Can you work these out from the model? Positions are in its coordinate system, mm. Face numbers are marked on the shaded views. A direction names the side the tool comes from. Round coordinates to 2 decimals unless told otherwise and drop trailing zeros. Write each loop counter-clockwise with the first axis right and the second up, starting at its lowest first coordinate (ties: lowest second). Pieces come first, ordered by that corner, then holes. Notation, with made-up numbers: (75.5, 79.25) - (124.5, 79.25) arc R16 ccw to (124.5, 99.25) - close; hole circle Ø11 at (57.25, -11). An arc over 180 degrees is marked (long way). One line per item, written item: value. Start each with the question number.
(1) I want a section at B-B on x = 2. List the corners of the cut face in (y, z) for me, plus the area to 3 significant figures.
(2) I want a section at D-D on x = 0. List the corners of the cut face in (y, z) for me, plus the area to 3 significant figures.
(3) I want a section at A-A on z = 4.5. List the corners of the cut face in (x, y) for me (3 decimals), plus the area to 3 significant figures.
(4) Thinking about a two-plate mould opening in Y: for the marked faces 1, 2, 3 and 4, which applies, +Y half, -Y half, draft (parallel to the pull), parting line (faces both ways), or undercut?
(5) I'm going to push flat-ended pins straight in: pin 1 Ø1 at (y, z) = (-5.5, 5) entering from -X; pin 2 Ø5 at (x, y) = (1.5, 4.5) entering from -Z. Where does each tip first touch, or does it pass through?
(6) I want a section at C-C on y = 4.5. List the corners of the cut face in (x, z) for me.
(7) On a 3-axis mill with a long thin cutter (end or side, diameter ignored), from which of +Z, -Z, +X, -X, +Y, -Y can I reach the whole of each face in a straight line? I mean the marked faces 5 and 6. Say none if no direction works.
(8) If I drill on L1, parallel to Y at x = -2.75, z = 2; L2, parallel to Y at x = 2.5, z = 3.5; L3, parallel to X at y = -7, z = 4, over which ranges is the centre line in solid material (lowest first)? Write a range as from..to.
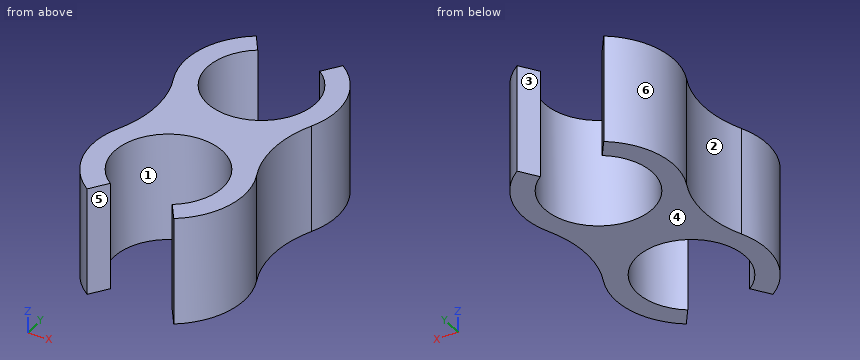
from build123d import *

# Parameters (mm, degrees)
F1_DEPTH = 6.35


with BuildPart() as f1:
    # F0 (on Top) → F1 (new body)
    with BuildSketch(Plane.XY):
        with BuildLine():
            ThreePointArc((1.821105, 7.045808), (0, 1.27), (-1.821105, 7.045808))
            Line((-1.821105, 7.045808), (-2.549547, 8.086131))
            ThreePointArc((-2.549547, 8.086131), (-4.286594, 5.621068), (-4.050685, 2.614706))
            ThreePointArc((-4.050685, 2.614706), (-3.487378, 0), (-4.050685, -2.614706))
            ThreePointArc((-4.050685, -2.614706), (-4.286594, -5.621068), (-2.549547, -8.086131))
            Line((-2.549547, -8.086131), (-1.821105, -7.045808))
            ThreePointArc((-1.821105, -7.045808), (0, -1.27), (1.821105, -7.045808))
            Line((1.821105, -7.045808), (2.549547, -8.086131))
            ThreePointArc((2.549547, -8.086131), (4.286594, -5.621068), (4.050685, -2.614706))
            ThreePointArc((4.050685, -2.614706), (3.487378, 0), (4.050685, 2.614706))
            ThreePointArc((4.050685, 2.614706), (4.286594, 5.621068), (2.549547, 8.086131))
            Line((2.549547, 8.086131), (1.821105, 7.045808))
        make_face()
    extrude(amount=F1_DEPTH)


solid = f1.part
Established:
1. outline: (-7.3, 0) - (-6.91, 0) - (-6.91, 6.35) - (-7.3, 6.35) - close; (-1.98, 0) - (1.98, 0) - (1.98, 6.35) - (-1.98, 6.35) - close; (6.91, 0) - (7.3, 0) - (7.3, 6.35) - (6.91, 6.35) - close
1. area: 30.1 mm2
2. outline: (-1.27, 0) - (1.27, 0) - (1.27, 6.35) - (-1.27, 6.35) - close
2. area: 16.1 mm2
3. outline: (-4.051, -2.615) arc R4.445 ccw to (-2.55, -8.086) - (-1.821, -7.046) arc R3.175 cw (long way) to (1.821, -7.046) - (2.55, -8.086) arc R4.445 ccw to (4.051, -2.615) arc R6.35 cw to (4.051, 2.615) arc R4.445 ccw to (2.55, 8.086) - (1.821, 7.046) arc R3.175 cw (long way) to (-1.821, 7.046) - (-2.55, 8.086) arc R4.445 ccw to (-4.051, 2.615) arc R6.35 cw to start
3. area: 56.9 mm2
4. face 1: undercut
4. face 2: undercut
4. face 3: +Y half
4. face 4: draft
5. pin 1: x = -4.41
5. pin 2: z = 0
6. outline: (-4.44, 0) - (-3.17, 0) - (-3.17, 6.35) - (-4.44, 6.35) - close; (3.17, 0) - (4.44, 0) - (4.44, 6.35) - (3.17, 6.35) - close
7. face 5: +Z, -Z, -Y
7. face 6: +Z, -Z, -X
8. L1: -7.94..-6.03, -2.86..2.86, 6.03..7.94
8. L2: -8.02..-6.4, -2.49..2.49, 6.4..8.02
8. L3: -3.64..-1.88, 1.88..3.64
